Read the model definition and answer for the solid it produces. Units are mm, in the model's axes. A direction names the side the tool comes from. Give positions to 0.01 mm unless a question says otherwise; leave off trailing zeros. Write each loop counter-clockwise with the first axis right and the second up, starting at its lowest first coordinate (ties: lowest second). Pieces come first, ordered by that corner, then holes. Notation, with made-up numbers: (-5, 28.25) -> (9, 28.25) arc R22 cw to (9, 52.25) -> close; hole circle Ø3 at (-13.75, 30). An arc over 180 degrees is marked (long way). Use a Markdown table: item, result.
from build123d import *

# Parameters (mm, degrees)
SKETCH_1_R          = 12.3
SKETCH_1_R_2        = 9
EXTRUDE_1_DEPTH     = 5
SKETCH_2_R          = 44
EXTRUDE_2_DEPTH     = 3
FILLET_1_R          = 3
CUT_EXTRUDE_1_DEPTH = 0.4


with BuildPart() as part:
    # Эскиз1 → Бобышка-Вытянуть1 (new body)
    with BuildSketch(Plane(origin=(0, 0, 0), x_dir=(1, 0, 0), z_dir=(0, 1, 0))):
        with Locations(Location((0, 0, 0), (0, 0, 270))):
            Circle(SKETCH_1_R)
        with Locations(Location((0, 0, 0), (0, 0, 270))):
            Circle(SKETCH_1_R_2, mode=Mode.SUBTRACT)
    extrude(amount=EXTRUDE_1_DEPTH)

    # Эскиз2 → Бобышка-Вытянуть2 (add)
    with BuildSketch(Plane.XZ):
        with Locations(Location((0, 0, 0), (0, 0, 270))):
            Circle(SKETCH_2_R)
    extrude(amount=EXTRUDE_2_DEPTH)

    # Скругление1
    fillet_1_edges = [part.edges().sort_by_distance(p)[0] for p in [
        (0, -3, 44),
    ]]
    fillet(fillet_1_edges, radius=FILLET_1_R - 0.0001)  # a hair under: the kernel refuses the full size

    # Эскиз3 → Вырез-Вытянуть1 (cut)
    with BuildSketch(Plane.XZ.offset(3)):
        with BuildLine():
            Line((8.995970712, -6.104573863), (15.540441866, -6.809702068))
            add(Edge.make_bspline(
                [(15.540441866, -6.809702068), (15.412468117, -7.209291312), (15.154055197, -8.016167909), (14.613314091, -9.189585554), (13.958158021, -10.343258865), (13.207970677, -11.497332402), (12.335909119, -12.632612277), (11.33678469, -13.743257832), (10.235946519, -14.845807978), (9.032648574, -15.91638665), (7.753536664, -16.930703687), (6.377129387, -17.80304501), (4.944504921, -18.539269968), (3.454192561, -19.15568009), (1.899553784, -19.624607238), (0.282665391, -19.970371161), (-1.395976393, -20.169412876), (-2.535298753, -20.19445388), (-3.112402685, -20.207137965)],
                knots=[0, 0, 0, 0, 0.821440156, 1.658705401, 2.525323128, 3.419405186, 4.353419828, 5.32681938, 6.344399772, 7.404443113, 8.481060479, 9.538977106, 10.591299887, 11.633537695, 12.694215778, 13.768160887, 14.869500701, 16, 16, 16, 16], degree=3))
            add(Edge.make_bspline(
                [(-3.112402685, -20.207137965), (-3.830059973, -20.180219947), (-5.24950882, -20.126979006), (-7.333765847, -19.748485297), (-9.324321869, -19.100876457), (-11.205038798, -18.21140963), (-12.947033456, -17.089230598), (-14.454993346, -15.681556769), (-15.775431133, -14.076428854), (-16.836564852, -12.230966933), (-17.674056128, -10.211434225), (-18.260978719, -8.036915844), (-18.637890858, -5.732029495), (-18.680542171, -4.148625261), (-18.702346595, -3.339149183)],
                knots=[0, 0, 0, 0, 0.998551589, 1.975027533, 2.936744805, 3.903838964, 4.863557655, 5.807675034, 6.763178998, 7.745855275, 8.758641806, 9.797744155, 10.874151411, 12, 12, 12, 12], degree=3))
            add(Edge.make_bspline(
                [(-18.702346595, -3.339149183), (-18.694827115, -2.798940969), (-18.679761602, -1.716616884), (-18.527910505, -0.102284621), (-18.301586091, 1.502865479), (-17.965102533, 3.090290283), (-17.549772791, 4.670349499), (-17.029049457, 6.231978524), (-16.419967141, 7.784615504), (-15.720819637, 9.310739002), (-14.951153945, 10.78597136), (-14.104651779, 12.165779349), (-13.228965259, 13.463701063), (-12.281997416, 14.653281312), (-11.271614555, 15.73843901), (-10.215647458, 16.72916995), (-9.109657465, 17.6327847), (-7.937840655, 18.421008283), (-6.733157575, 19.121726424), (-5.503022782, 19.73623986), (-4.241088179, 20.242359886), (-2.95541361, 20.657688994), (-1.650714865, 20.995350946), (-0.320069938, 21.221805432), (1.034040545, 21.37348169), (1.947944187, 21.388084339), (2.407429046, 21.395426137)],
                knots=[0, 0, 0, 0, 1.075906032, 2.155611451, 3.227554832, 4.30373447, 5.38628686, 6.480642286, 7.581143633, 8.707391042, 9.82337293, 10.893692135, 11.930684225, 12.940768785, 13.919223559, 14.881988069, 15.823529777, 16.761054785, 17.692163021, 18.598508727, 19.497917784, 20.397951545, 21.288749041, 22.180057169, 23.084984307, 24, 24, 24, 24], degree=3))
            add(Edge.make_bspline(
                [(2.407429046, 21.395426137), (2.984709253, 21.38436262), (4.110243009, 21.362791879), (5.755422445, 21.146858145), (7.309280074, 20.798674498), (8.776183147, 20.306894686), (10.163630571, 19.698295383), (11.445405048, 18.914546867), (12.642602428, 18.007561118), (13.744215102, 16.970925789), (14.740391422, 15.815186826), (15.5940589, 14.539264454), (16.346732625, 13.178856469), (16.935563309, 11.70304546), (17.399883233, 10.131680694), (17.72749797, 8.457159294), (17.928240109, 6.684462125), (17.952122631, 5.468151048), (17.964320071, 4.846948573)],
                knots=[0, 0, 0, 0, 1.079196217, 2.10412856, 3.097265039, 4.052997914, 4.993829394, 5.924450447, 6.855882321, 7.798592485, 8.748507102, 9.702980304, 10.665060364, 11.651045023, 12.668191174, 13.725659051, 14.838433479, 16, 16, 16, 16], degree=3))
            add(Edge.make_bspline(
                [(17.964320071, 4.846948573), (17.939861422, 3.857360897), (17.890041697, 1.84167366), (17.596116304, -0.153181552), (17.446491546, -1.168676427)],
                knots=[0, 0, 0, 0, 0.981886135, 2, 2, 2, 2], degree=3))
            Line((17.446491546, -1.168676427), (-11.651064544, -1.168676427))
            add(Edge.make_bspline(
                [(-11.651064544, -1.168676427), (-11.757884651, -1.36504795), (-11.95927427, -1.735270255), (-12.188010225, -2.298230913), (-12.326177646, -2.83296849), (-12.346562226, -3.184220667), (-12.356192749, -3.350166811)],
                knots=[0, 0, 0, 0, 1.156942796, 2.181202349, 3.140724307, 4, 4, 4, 4], degree=3))
            add(Edge.make_bspline(
                [(-12.356192749, -3.350166811), (-12.34747649, -3.820530136), (-12.330558483, -4.733491811), (-12.207588937, -6.058525833), (-12.012779093, -7.30055293), (-11.73295496, -8.457242596), (-11.349108398, -9.521277255), (-10.912446511, -10.511594722), (-10.387891199, -11.419433456), (-9.762517234, -12.22046917), (-9.095103061, -12.940939566), (-8.37345163, -13.553599554), (-7.633662355, -14.094798444), (-6.845003469, -14.527977227), (-6.01676525, -14.853496387), (-5.158998119, -15.10327405), (-4.2632374, -15.248645974), (-3.652782517, -15.263647049), (-3.343772877, -15.271240529)],
                knots=[0, 0, 0, 0, 1.346284225, 2.613098929, 3.805631801, 4.942804233, 6.013450698, 7.039235158, 8.038108926, 9.00533571, 9.942442562, 10.84439418, 11.710848438, 12.56244313, 13.41163356, 14.253504373, 15.115931414, 16, 16, 16, 16], degree=3))
            add(Edge.make_bspline(
                [(-3.343772877, -15.271240529), (-2.749342022, -15.245702869), (-1.550628193, -15.194204288), (0.219580647, -14.702324431), (1.984521743, -13.976401138), (3.39348022, -13.111143469), (4.503332391, -12.310342129), (5.279497704, -11.607205665), (6.028705195, -10.857717747), (6.714675872, -10.028152313), (7.372080008, -9.148002655), (7.963425509, -8.192752467), (8.520742644, -7.181562683), (8.836014409, -6.467075917), (8.995970712, -6.104573863)],
                knots=[0, 0, 0, 0, 1.313044299, 2.647851039, 4.03980324, 5.527339259, 6.29475363, 7.066375866, 7.842396062, 8.63863277, 9.446691243, 10.272184996, 11.123375662, 12, 12, 12, 12], degree=3))
        make_face()
        with BuildLine():
            Line((-10.57133698, 3.767221009), (11.585113341, 3.767221009))
            add(Edge.make_bspline(
                [(11.585113341, 3.767221009), (11.593025495, 4.083048202), (11.606273104, 4.611849202), (11.614751545, 5.140746771), (11.618166225, 5.353759471)],
                knots=[0, 0, 0, 0, 1.194503009, 2, 2, 2, 2], degree=3))
            add(Edge.make_bspline(
                [(11.618166225, 5.353759471), (11.607865414, 5.787266581), (11.587754302, 6.633637755), (11.485258286, 7.865088987), (11.282712763, 9.016930024), (11.014497534, 10.093427235), (10.643340787, 11.084224083), (10.22296171, 12.00905194), (9.693440715, 12.841121184), (9.10342503, 13.5981791), (8.450495006, 14.275095215), (7.747736216, 14.858424007), (6.995642953, 15.349517378), (6.205542288, 15.762387273), (5.357586525, 16.065155124), (4.475125766, 16.303564325), (3.542488324, 16.434420376), (2.907267946, 16.451055439), (2.583711097, 16.459528702)],
                knots=[0, 0, 0, 0, 1.288915635, 2.516454775, 3.668675548, 4.762204166, 5.808675246, 6.809806692, 7.776046417, 8.732555008, 9.659000055, 10.566141369, 11.441184925, 12.324901883, 13.209090714, 14.112018255, 15.038334656, 16, 16, 16, 16], degree=3))
            add(Edge.make_bspline(
                [(2.583711097, 16.459528702), (2.226745831, 16.453545839), (1.52033684, 16.441706179), (0.475354062, 16.270793025), (-0.551481717, 16.041052654), (-1.545895478, 15.676402937), (-2.521085999, 15.236321875), (-3.474458828, 14.69783397), (-4.385955956, 14.033830496), (-5.29217066, 13.304160782), (-6.156416477, 12.463653114), (-6.953362323, 11.511724736), (-7.714463763, 10.47410691), (-8.384666445, 9.319187587), (-9.037211223, 8.085112247), (-9.596912384, 6.732446378), (-10.136432386, 5.293123636), (-10.424137331, 4.283684469), (-10.57133698, 3.767221009)],
                knots=[0, 0, 0, 0, 0.867869597, 1.717452491, 2.571772394, 3.425671253, 4.289803496, 5.174634535, 6.084973587, 7.031591473, 8.005136717, 9.013559597, 10.050697067, 11.133079613, 12.260592687, 13.446148552, 14.693362615, 16, 16, 16, 16], degree=3))
        make_face(mode=Mode.SUBTRACT)
    extrude(amount=-CUT_EXTRUDE_1_DEPTH, mode=Mode.SUBTRACT)


solid = part.part
Item 1: Straight lines are drawn through the part: line 1 along X through (y, z) = (1.5, 0); line 2 along Y through (x, z) = (-13, 13.5); line 3 along Y through (x, z) = (-21.5, 21.5). For each, find the intervals that lie inside material, in ascending order. Write a range as [from, to].
Return value:
| item | result |
|---|---|
| line 1 | [-12.3, -9], [9, 12.3] |
| line 2 | [-2.6, 0] |
| line 3 | [-3, 0] |
Item 2: For a pull along X with two mould halves and no side action, classify faces 3 (the face through (-12, 2.5, -2.7)), 4 (the face through (2.703, 2.465, 8.584)), 5 (the face through (-9, 0, -9)), 6 (the face through (0, -2.6, 1)) as +X half, -X half, draft (parallel to the pull), parting line (faces both ways), or undercut.
Return value:
| item | result |
|---|---|
| face 3 | parting line |
| face 4 | undercut |
| face 5 | draft |
| face 6 | undercut |
Item 3: A tool of negligible diameter and unlimited length cuts with its end or side. For faces 1 (the face through (0, 0, 0)), 2 (the face through (1, -3, 9)), from which of +Z, -Z, +X, -X, +Y, -Y can it reach the whole face along a straight path? Write none if from no direction.
Return value:
| item | result |
|---|---|
| face 1 | +Y |
| face 2 | +Z, -Z, +X, -X, -Y |
Item 4: A cutting plane is placed at A-A (y = 3). Give the vertices of the cut face in (x, z).
Return value:
| item | result |
|---|---|
| outline | circle Ø24.6 at (0, 0); hole circle Ø18 at (0, 0) |
Item 5: Each of these flat-tipped pins is pushed along its axis until it touches: P1, Ø2, axis at x = 5.5, y = 3, coming from the +Z side; P2, Ø8, axis at x = -32, z = 16.5, coming from the +Y side; P3, Ø2, axis at x = -27.5, y = -2, coming from the -Z side. Where does it stop, or does it pass through?
Return value:
| item | result |
|---|---|
| P1 | z = 11.45 |
| P2 | y = 0 |
| P3 | z = -34.54 |
